Can you work these out from the model? Positions are in its coordinate system, mm. A direction names the side the tool comes from. Coordinates: 2 decimals unless noted, no trailing zeros. Loops run counter-clockwise (first coordinate to the right, second up) from the corner with the lowest first, then second, coordinate; pieces in that order, holes last. Notation, with made-up numbers: M -35,-24 L 11,-24 A15 ccw 11,-20 Z; hole C 2,0 d5. An arc over 180 degrees is marked long. Answer as a JSON object with one key per item and string values. Group by question number.
Item 1: If I drill on line 1 (Z direction, x = 30, y = -3.25); line 2 (X direction, y = -4.25, z = 6); line 3 (X direction, y = -0.75, z = -21), over which ranges is the centre line in solid material (lowest first)?
Item 2: We'd pull the mould along X, two halves only. Please class faces 1 (the flat face through (-26, -3, -14.444)), 2 (the flat face through (-149.778, -3, 6)), 3 (the flat face through (-3, 0, -22)), 4 (the cylindrical face through (5.42, -1.08, 31.06)): +X half, -X half, draft (parallel to the pull), parting line (faces both ways), or undercut.
Item 3: Suppose I cut it at A-A (x = 30.5). Write out the boundary of the cut face in (y, z).
Item 4: Which directions (+Z, -Z, +X, -X, +Y, -Y) give clear straight access to the entire face, cutting with the end or side of a thin tool? Please do faces 5 (the flat face through (-28, -3, 25.556)), 6 (the flat face through (-3.3, -6.35, -21.7)).
Item 5: I'm going to push flat-ended pins straight in: pin 1 Ø8 at (x, z) = (-44.78, -24.44) entering from +Y; pin 2 Ø10.5 at (x, z) = (5.22, -24.44) entering from -Y; pin 3 Ø14.5 at (x, z) = (-44.78, 35.56) entering from -Y. Where does each tip first touch, or does it pass through?
Item 6: Suppose I cut it at B-B (y = -4). Count the separate pieces of the cut face and the enclosed holes in it, then the cut area to 3 significant figures.
Item 7: Suppose I cut it at C-C (z = 0.5). Write out the boundary of the cut face in (x, y), then the cut area to 3 significant figures.
```python
from build123d import *

# Parameters (mm, degrees)
CROQUIS1_W                                      = 297.15
CROQUIS1_H                                      = 80
BRIDA_BASE1_DEPTH                               = 6.35
REDONDEO1_R                                     = 2
TALADRO_DE_MARGEN_PARA_M51_D                    = 5.5
CROQUIS9_R                                      = 20
CORTAR_EXTRUIR1_DEPTH                           = 10
CSK_FOR_M8_OVAL_HEAD_MACHINE_SCREW1_D           = 9
CSK_FOR_M8_OVAL_HEAD_MACHINE_SCREW1_CSINK_D     = 17.3
CSK_FOR_M8_OVAL_HEAD_MACHINE_SCREW1_CSINK_ANGLE = 90


# Sheet-metal steps are written as plain solids
with BuildPart() as part:
    # Croquis1 → Brida base1 (new body)
    with BuildSketch(Plane(origin=(0, 0, 0), x_dir=(1, 0, 0), z_dir=(0, 1, 0))):
        with Locations((-1.202777778, -5.555555556)):
            Rectangle(CROQUIS1_W, CROQUIS1_H)
    extrude(amount=-BRIDA_BASE1_DEPTH)

    # Redondeo1
    redondeo1_edges = [part.edges().sort_by_distance(p)[0] for p in [
        (-149.777777778, -3.175, -34.444444444),
        (-149.777777778, -3.175, 45.555555556),
    ]]
    fillet(redondeo1_edges, radius=REDONDEO1_R)

    # Taladro de margen para M51 (through all)
    with Locations(Plane(origin=(0, 0, 0), x_dir=(1, 0, 0), z_dir=(0, 1, 0))):
        with Locations((-119.777777778, 24.444444444), (-119.777777778, -35.555555556), (80.222222222, -35.555555556), (80.222222222, 24.444444444)):
            Hole(TALADRO_DE_MARGEN_PARA_M51_D / 2)

    # Croquis9 → Cortar-Extruir1 (cut)
    with BuildSketch(Plane(origin=(0, -6.35, 0), x_dir=(-1, 0, 0), z_dir=(0, -1, 0))):
        with Locations(Location((-104.209895864, -5.555555556, 0), (0, 0, 90))):
            Circle(CROQUIS9_R)
        with BuildLine():
            Line((-41.389105309, 14.444444444), (95.628093505, 14.444444444))
            ThreePointArc((95.628093505, 14.444444444), (115.628093505, -5.555555556), (95.628093505, -25.555555556))
            Line((95.628093505, -25.555555556), (-41.389105309, -25.555555556))
            ThreePointArc((-41.389105309, -25.555555556), (-61.389105309, -5.555555556), (-41.389105309, 14.444444444))
        make_face()
    extrude(amount=-CORTAR_EXTRUIR1_DEPTH, mode=Mode.SUBTRACT)

    # CSK for M8 Oval Head Machine Screw1 (through all)
    with Locations(Plane(origin=(-44.777777778, -6.35, -24.444444444), x_dir=(0, 0, -1), z_dir=(0, -1, 0))):
        with Locations((0, 0), (0, 50), (-60, 50), (-60, 0)):
            CounterSinkHole(CSK_FOR_M8_OVAL_HEAD_MACHINE_SCREW1_D / 2, CSK_FOR_M8_OVAL_HEAD_MACHINE_SCREW1_CSINK_D / 2, counter_sink_angle=CSK_FOR_M8_OVAL_HEAD_MACHINE_SCREW1_CSINK_ANGLE)


solid = part.part
```
From the geometry:
{
 "1": {"line 1": "-34.44 to -14.44, 25.56 to 45.56", "line 2": "-149.78 to -115.62, 61.38 to 84.21, 124.2 to 147.37", "line 3": "-149.78 to -47.67, -41.88 to 2.33, 8.12 to 147.37"},
 "2": {"face 1": "undercut", "face 2": "-X half", "face 3": "draft", "face 4": "undercut"},
 "3": {"outline": "M -6.35,-34.44 L 0,-34.44 L 0,-14.44 L -6.35,-14.44 Z; M -6.35,25.56 L 0,25.56 L 0,45.56 L -6.35,45.56 Z"},
 "4": {"face 5": "+Y, -Y", "face 6": "+Z, -Z, +X, -X, -Y"},
 "5": {"pin 1": "through", "pin 2": "y = -2.95", "pin 3": "y = -4.95"},
 "6": {"separate pieces": "1", "enclosed holes": "10", "area": "15,200 mm2"},
 "7": {"outline": "M -149.78,-6.35 L -114.98,-6.35 L -114.98,0 L -149.78,0 Z; M 60.74,-6.35 L 84.86,-6.35 L 84.86,0 L 60.74,0 Z; M 123.56,-6.35 L 147.37,-6.35 L 147.37,0 L 123.56,0 Z", "area": "525 mm2"}
}
